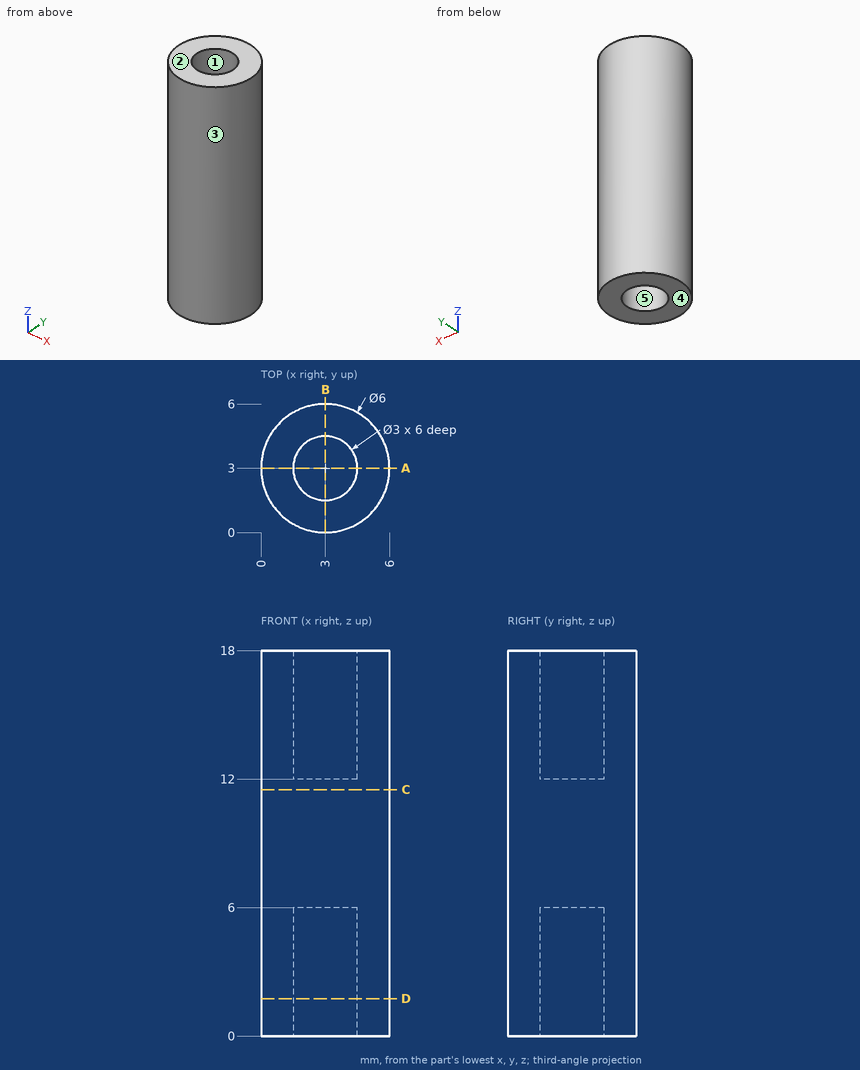
Could you check a few things on this drawing? It's one solid part, dimensions in mm from its lowest x, y, z. A direction names the side the tool comes from. Round coordinates to 2 decimals unless told otherwise and drop trailing zeros. Write each loop counter-clockwise with the first axis right and the second up, starting at its lowest first coordinate (ties: lowest second). Pieces come first, ordered by that corner, then holes. Notation, with made-up numbers: (63.5, 32) -> (78.5, 32) arc R29 ccw to (78.5, 64) -> close; hole circle Ø9 at (86.5, 32). An arc over 180 degrees is marked (long way). One line per item, written item: value.
1) I'm going to push flat-ended pins straight in: pin 1 Ø2 at (y, z) = (5, 2.5) entering from -X; pin 2 Ø1.5 at (x, y) = (3.5, 3) entering from +Z; pin 3 Ø1.5 at (x, y) = (3, 3.5) entering from -Z. Where does each tip first touch, or does it pass through?
Filled sheet:
pin 1: stops at x = 0.17
pin 2: stops at z = 12
pin 3: stops at z = 6
2) Suppose I cut it at C-C on z = 11.5. List the corners of the cut face in (x, y) for me.
Filled sheet:
outline: circle Ø6 at (3, 3)
3) Suppose I cut it at D-D on z = 1.75. List the corners of the cut face in (x, y) for me.
Filled sheet:
outline: circle Ø6 at (3, 3); hole circle Ø3 at (3, 3)
4) If I drill on line 1 (Y direction, x = 3.1, z = 12.75); line 2 (Y direction, x = 3.1, z = 9), over which ranges is the centre line in solid material (lowest first)? Write a range as [from, to].
Filled sheet:
line 1: y = [0, 1.5], [4.5, 6]
line 2: y = [0, 6]
5) We'd pull the mould along X, two halves only. Please class the marked faces 3, 4 and 5: released by +X, released by -X, zero draft, split by the parting line, or undercut.
Filled sheet:
face 3: split by the parting line
face 4: zero draft
face 5: undercut
6) Suppose I cut it at A-A on y = 3. List the corners of the cut face in (x, z) for me, plus the area to 3 significant figures.
Filled sheet:
outline: (0, 0) -> (1.5, 0) -> (1.5, 6) -> (4.5, 6) -> (4.5, 0) -> (6, 0) -> (6, 18) -> (4.5, 18) -> (4.5, 12) -> (1.5, 12) -> (1.5, 18) -> (0, 18) -> close
area: 72.0 mm2
7) For the marked faces 1 and 2, which set-ups out of +Z, -Z, +X, -X, +Y, -Y let a thin tool reach every point of the face, with its end or its side?
Filled sheet:
face 1: +Z
face 2: +Z, +X, -X, +Y, -Y
